Design review of the part built by this model. Coordinates are the model's own, in mm. A direction names the side the tool comes from. Give positions to 0.01 mm unless a question says otherwise; leave off trailing zeros. Write each loop counter-clockwise with the first axis right and the second up, starting at its lowest first coordinate (ties: lowest second). Pieces come first, ordered by that corner, then holes. Notation, with made-up numbers: (81.5, 33.5) -> (87.5, 33.5) arc R25 cw to (87.5, 46.5) -> close; hole circle Ø10 at (33, 35). An arc over 180 degrees is marked (long way). Put each result on its own line as item: value. Start each with the question number.
from build123d import *

# Parameters (mm, degrees)
CROQUIS3_R                = 2.5
PG20_T_SLOT_20X20_1_DEPTH = 232.5


with BuildPart() as part:
    # Croquis3 → Pg20_t_slot 20X20(1) (new body)
    with BuildSketch(Plane.XY):
        with BuildLine():
            Line((-2.218019485, 3.9), (2.218019485, 3.9))
            ThreePointArc((2.218019485, 3.9), (2.792044633, 4.014180701), (3.278679656, 4.339339828))
            Line((3.278679656, 4.339339828), (5.417989899, 6.478650071))
            ThreePointArc((5.417989899, 6.478650071), (5.478686269, 6.569488608), (5.5, 6.676639969))
            Line((5.5, 6.676639969), (5.5, 7.92))
            ThreePointArc((5.5, 7.92), (5.417989899, 8.117989899), (5.22, 8.2))
            Line((5.22, 8.2), (3.38, 8.2))
            ThreePointArc((3.38, 8.2), (3.182010101, 8.282010101), (3.1, 8.48))
            Line((3.1, 8.48), (3.1, 9.42))
            ThreePointArc((3.1, 9.42), (3.182010101, 9.617989899), (3.38, 9.7))
            Line((3.38, 9.7), (3.6, 9.7))
            Line((3.6, 9.7), (3.6, 9.72))
            ThreePointArc((3.6, 9.72), (3.682010101, 9.917989899), (3.88, 10))
            Line((3.88, 10), (8.5, 10))
            ThreePointArc((8.5, 10), (9.560660172, 9.560660172), (10, 8.5))
            Line((10, 8.5), (10, 3.88))
            ThreePointArc((10, 3.88), (9.917989899, 3.682010101), (9.72, 3.6))
            Line((9.72, 3.6), (9.7, 3.6))
            Line((9.7, 3.6), (9.7, 3.38))
            ThreePointArc((9.7, 3.38), (9.617989899, 3.182010101), (9.42, 3.1))
            Line((9.42, 3.1), (8.48, 3.1))
            ThreePointArc((8.48, 3.1), (8.282010101, 3.182010101), (8.2, 3.38))
            Line((8.2, 3.38), (8.2, 5.22))
            ThreePointArc((8.2, 5.22), (8.117989899, 5.417989899), (7.92, 5.5))
            Line((7.92, 5.5), (6.676639969, 5.5))
            ThreePointArc((6.676639969, 5.5), (6.569488608, 5.478686269), (6.478650071, 5.417989899))
            Line((6.478650071, 5.417989899), (4.339339828, 3.278679656))
            ThreePointArc((4.339339828, 3.278679656), (4.014180701, 2.792044633), (3.9, 2.218019485))
            Line((3.9, 2.218019485), (3.9, -2.218019485))
            ThreePointArc((3.9, -2.218019485), (4.014180701, -2.792044633), (4.339339828, -3.278679656))
            Line((4.339339828, -3.278679656), (6.478650071, -5.417989899))
            ThreePointArc((6.478650071, -5.417989899), (6.569488608, -5.478686269), (6.676639969, -5.5))
            Line((6.676639969, -5.5), (7.92, -5.5))
            ThreePointArc((7.92, -5.5), (8.117989899, -5.417989899), (8.2, -5.22))
            Line((8.2, -5.22), (8.2, -3.38))
            ThreePointArc((8.2, -3.38), (8.282010101, -3.182010101), (8.48, -3.1))
            Line((8.48, -3.1), (9.42, -3.1))
            ThreePointArc((9.42, -3.1), (9.617989899, -3.182010101), (9.7, -3.38))
            Line((9.7, -3.38), (9.7, -3.6))
            Line((9.7, -3.6), (9.72, -3.6))
            ThreePointArc((9.72, -3.6), (9.917989899, -3.682010101), (10, -3.88))
            Line((10, -3.88), (10, -8.5))
            ThreePointArc((10, -8.5), (9.560660172, -9.560660172), (8.5, -10))
            Line((8.5, -10), (3.88, -10))
            ThreePointArc((3.88, -10), (3.682010101, -9.917989899), (3.6, -9.72))
            Line((3.6, -9.72), (3.6, -9.7))
            Line((3.6, -9.7), (3.38, -9.7))
            ThreePointArc((3.38, -9.7), (3.182010101, -9.617989899), (3.1, -9.42))
            Line((3.1, -9.42), (3.1, -8.48))
            ThreePointArc((3.1, -8.48), (3.182010101, -8.282010101), (3.38, -8.2))
            Line((3.38, -8.2), (5.22, -8.2))
            ThreePointArc((5.22, -8.2), (5.417989899, -8.117989899), (5.5, -7.92))
            Line((5.5, -7.92), (5.5, -6.676639969))
            ThreePointArc((5.5, -6.676639969), (5.478686269, -6.569488608), (5.417989899, -6.478650071))
            Line((5.417989899, -6.478650071), (3.278679656, -4.339339828))
            ThreePointArc((3.278679656, -4.339339828), (2.792044633, -4.014180701), (2.218019485, -3.9))
            Line((2.218019485, -3.9), (-2.218019485, -3.9))
            ThreePointArc((-2.218019485, -3.9), (-2.792044633, -4.014180701), (-3.278679656, -4.339339828))
            Line((-3.278679656, -4.339339828), (-5.417989899, -6.478650071))
            ThreePointArc((-5.417989899, -6.478650071), (-5.478686269, -6.569488608), (-5.5, -6.676639969))
            Line((-5.5, -6.676639969), (-5.5, -7.92))
            ThreePointArc((-5.5, -7.92), (-5.417989899, -8.117989899), (-5.22, -8.2))
            Line((-5.22, -8.2), (-3.38, -8.2))
            ThreePointArc((-3.38, -8.2), (-3.182010101, -8.282010101), (-3.1, -8.48))
            Line((-3.1, -8.48), (-3.1, -9.42))
            ThreePointArc((-3.1, -9.42), (-3.182010101, -9.617989899), (-3.38, -9.7))
            Line((-3.38, -9.7), (-3.6, -9.7))
            Line((-3.6, -9.7), (-3.6, -9.72))
            ThreePointArc((-3.6, -9.72), (-3.682010101, -9.917989899), (-3.88, -10))
            Line((-3.88, -10), (-8.5, -10))
            ThreePointArc((-8.5, -10), (-9.560660172, -9.560660172), (-10, -8.5))
            Line((-10, -8.5), (-10, -3.88))
            ThreePointArc((-10, -3.88), (-9.917989899, -3.682010101), (-9.72, -3.6))
            Line((-9.72, -3.6), (-9.7, -3.6))
            Line((-9.7, -3.6), (-9.7, -3.38))
            ThreePointArc((-9.7, -3.38), (-9.617989899, -3.182010101), (-9.42, -3.1))
            Line((-9.42, -3.1), (-8.48, -3.1))
            ThreePointArc((-8.48, -3.1), (-8.282010101, -3.182010101), (-8.2, -3.38))
            Line((-8.2, -3.38), (-8.2, -5.22))
            ThreePointArc((-8.2, -5.22), (-8.117989899, -5.417989899), (-7.92, -5.5))
            Line((-7.92, -5.5), (-6.676639969, -5.5))
            ThreePointArc((-6.676639969, -5.5), (-6.569488608, -5.478686269), (-6.478650071, -5.417989899))
            Line((-6.478650071, -5.417989899), (-4.339339828, -3.278679656))
            ThreePointArc((-4.339339828, -3.278679656), (-4.014180701, -2.792044633), (-3.9, -2.218019485))
            Line((-3.9, -2.218019485), (-3.9, 2.218019485))
            ThreePointArc((-3.9, 2.218019485), (-4.014180701, 2.792044633), (-4.339339828, 3.278679656))
            Line((-4.339339828, 3.278679656), (-6.478650071, 5.417989899))
            ThreePointArc((-6.478650071, 5.417989899), (-6.569488608, 5.478686269), (-6.676639969, 5.5))
            Line((-6.676639969, 5.5), (-7.92, 5.5))
            ThreePointArc((-7.92, 5.5), (-8.117989899, 5.417989899), (-8.2, 5.22))
            Line((-8.2, 5.22), (-8.2, 3.38))
            ThreePointArc((-8.2, 3.38), (-8.282010101, 3.182010101), (-8.48, 3.1))
            Line((-8.48, 3.1), (-9.42, 3.1))
            ThreePointArc((-9.42, 3.1), (-9.617989899, 3.182010101), (-9.7, 3.38))
            Line((-9.7, 3.38), (-9.7, 3.6))
            Line((-9.7, 3.6), (-9.72, 3.6))
            ThreePointArc((-9.72, 3.6), (-9.917989899, 3.682010101), (-10, 3.88))
            Line((-10, 3.88), (-10, 8.5))
            ThreePointArc((-10, 8.5), (-9.560660172, 9.560660172), (-8.5, 10))
            Line((-8.5, 10), (-3.88, 10))
            ThreePointArc((-3.88, 10), (-3.682010101, 9.917989899), (-3.6, 9.72))
            Line((-3.6, 9.72), (-3.6, 9.7))
            Line((-3.6, 9.7), (-3.38, 9.7))
            ThreePointArc((-3.38, 9.7), (-3.182010101, 9.617989899), (-3.1, 9.42))
            Line((-3.1, 9.42), (-3.1, 8.48))
            ThreePointArc((-3.1, 8.48), (-3.182010101, 8.282010101), (-3.38, 8.2))
            Line((-3.38, 8.2), (-5.22, 8.2))
            ThreePointArc((-5.22, 8.2), (-5.417989899, 8.117989899), (-5.5, 7.92))
            Line((-5.5, 7.92), (-5.5, 6.676639969))
            ThreePointArc((-5.5, 6.676639969), (-5.478686269, 6.569488608), (-5.417989899, 6.478650071))
            Line((-5.417989899, 6.478650071), (-3.278679656, 4.339339828))
            ThreePointArc((-3.278679656, 4.339339828), (-2.792044633, 4.014180701), (-2.218019485, 3.9))
        make_face()
        Circle(CROQUIS3_R, mode=Mode.SUBTRACT)
    extrude(amount=PG20_T_SLOT_20X20_1_DEPTH)


solid = part.part
Q1. To check wall thickness, follow probe 1 along X at (y, z) = (-3.25, 15.5); probe 2 along Y at (x, z) = (0, 88.5). State the ranges of each line that lie inside material, in increasing order. Write a range as from..to.
Q2. For pin 1 (0.5 mm diameter, centred on x = 9, z = 149.5, fed in from +Y); pin 2 (5 mm diameter, centred on x = 1, z = 83, fed in from +Y); pin 3 (0.5 mm diameter, centred on y = -9, z = 124.5, fed in from +X), all flat-tipped, find the tip position at first contact; note any pin that passes through.
Q3. Take a section at A-A on y = 0. Give the boundary of the cut face in (x, z), then the cut area to 3 significant figures.
Q4. Mouldability with a two-part tool opening along Y and no side actions: class faces 1 (the face through (3.9, 0, 115)), 2 (the face through (-6, 10, 115)), 3 (the face through (-10, 6, 115)) as +Y half, -Y half, draft (parallel to the pull), parting line (faces both ways), or undercut.
Q5. Machinability: for faces 4 (the face through (10, -6, 115)), 5 (the face through (-3.9, 0, 115)), 6 (the face through (0, -3.9, 115)), 7 (the face through (0, 3.9, 115)), which of the approach directions +Z, -Z, +X, -X, +Y, -Y give a long, thin tool a straight path to every point of the face, cutting with its end or side? Answer none if there is none.
Result:
1. probe 1: x = -9.67..-8.23, -4.31..4.31, 8.23..9.67
1. probe 2: y = -3.9..-2.5, 2.5..3.9
2. pin 1: stops at y = 9.98
2. pin 2: stops at y = 9.7
2. pin 3: stops at x = 9.98
3. outline: (-3.9, 0) -> (-2.5, 0) -> (-2.5, 232.5) -> (-3.9, 232.5) -> close; (2.5, 0) -> (3.9, 0) -> (3.9, 232.5) -> (2.5, 232.5) -> close
3. area: 651 mm^2
4. face 1: undercut
4. face 2: +Y half
4. face 3: draft
5. face 4: +Z, -Z, +X, +Y, -Y
5. face 5: +Z, -Z, -X
5. face 6: +Z, -Z, -Y
5. face 7: +Z, -Z, +Y
